CAD build for the part. Positions are in the model's coordinates, mm. A direction names the side the tool comes from. Give positions to 0.01 mm unless a question says otherwise; leave off trailing zeros. Loops run counter-clockwise (first coordinate to the right, second up) from the corner with the lowest first, then second, coordinate; pieces in that order, holes last. Notation, with made-up numbers: (74, 30.25) - (114, 30.25) arc R28 cw to (114, 50.25) - close; hole circle Ø11 at (51.5, 25.25). An arc over 180 degrees is marked (long way). Return JSON: item names as keys, results as strings.
from build123d import *

# Parameters (mm, degrees)
SKETCH1_W           = 220
SKETCH1_H           = 220
BOSS_EXTRUDE1_DEPTH = 4.5
SKETCH2_W           = 220
SKETCH2_H           = 135
BOSS_EXTRUDE2_DEPTH = 4
SKETCH3_W           = 150
SKETCH3_H           = 75
BOSS_EXTRUDE3_DEPTH = 45
SKETCH4_W           = 170
SKETCH4_H           = 110
BOSS_EXTRUDE4_DEPTH = 45
SKETCH5_W           = 280
SKETCH5_H           = 220
BOSS_EXTRUDE5_DEPTH = 4.5
SKETCH6_R           = 1.5
CUT_EXTRUDE1_DEPTH  = 10


with BuildPart() as part:
    # Sketch1 → Boss-Extrude1 (new body)
    with BuildSketch(Plane(origin=(0, 0, 0), x_dir=(1, 0, 0), z_dir=(0, 1, 0))):
        with Locations((-18.301886792, -38.490566038)):
            Rectangle(SKETCH1_W, SKETCH1_H)
    extrude(amount=BOSS_EXTRUDE1_DEPTH)

    # Sketch2 → Boss-Extrude2 (add)
    with BuildSketch(Plane(origin=(0, 4.5, 0), x_dir=(1, 0, 0), z_dir=(0, 1, 0))):
        with Locations((-18.301886792, -65.990566038)):
            Rectangle(SKETCH2_W, SKETCH2_H)
    extrude(amount=BOSS_EXTRUDE2_DEPTH)

    # Sketch3 → Boss-Extrude3 (add)
    with BuildSketch(Plane(origin=(0, 4.5, 0), x_dir=(1, 0, 0), z_dir=(0, 1, 0))):
        with Locations((16.698113208, 34.009433962)):
            Rectangle(SKETCH3_W, SKETCH3_H)
    extrude(amount=BOSS_EXTRUDE3_DEPTH)

    # Sketch4 → Boss-Extrude4 (add)
    with BuildSketch(Plane(origin=(0, 8.5, 0), x_dir=(1, 0, 0), z_dir=(0, 1, 0))):
        with Locations((6.698113208, -63.490566038)):
            Rectangle(SKETCH4_W, SKETCH4_H)
    extrude(amount=BOSS_EXTRUDE4_DEPTH)

    # Sketch5 → Boss-Extrude5 (add)
    with BuildSketch(Plane.XZ):
        with Locations((-48.301886792, 38.490566038)):
            Rectangle(SKETCH5_W, SKETCH5_H)
    extrude(amount=BOSS_EXTRUDE5_DEPTH)

    # Sketch6 → Cut-Extrude1 (cut)
    with BuildSketch(Plane(origin=(0, 0, 0), x_dir=(1, 0, 0), z_dir=(0, 1, 0))):
        with Locations(Location((-168.301886792, 61.509433962, 0), (0, 0, 270))):
            Circle(SKETCH6_R)
        with Locations(Location((-168.301886792, -138.490566038, 0), (0, 0, 270))):
            Circle(SKETCH6_R)
    extrude(amount=-CUT_EXTRUDE1_DEPTH, mode=Mode.SUBTRACT)


solid = part.part
1. Cut at C-C, the plane x = -17.5. Write the cut outline in (y, z).
Values follow:
{"outline": "(-4.5, -71.51) - (49.5, -71.51) - (49.5, 3.49) - (8.5, 3.49) - (8.5, 8.49) - (53.5, 8.49) - (53.5, 118.49) - (8.5, 118.49) - (8.5, 133.49) - (4.5, 133.49) - (4.5, 148.49) - (-4.5, 148.49) - close"}
2. Which spindle directions (+Z, -Z, +X, -X, +Y, -Y) get a long thin tool onto all of the face, cutting with end or side? Do faces 1 (the face through (16, 49.5, -35)), 2 (the face through (-94, 4.5, -37)), 3 (the face through (-128.302, 3, 40)). Say none if no direction does.
Values follow:
{"face 1": "-Z, +X, -X, +Y", "face 2": "-Z, -X, +Y", "face 3": "+Z, -Z, -X, +Y"}
3. Drop flat-ended pins along their axis: P1, Ø4, axis at y = 33.5, z = 111.5, coming from the -X side; P2, Ø6, axis at x = 22, y = 28.5, coming from the +Z side; P3, Ø3.5, axis at x = -168.3, z = 138.49, coming from the +Y side; P4, Ø2.5, axis at x = -168.3, z = -61.51, coming from the -Y side. Give the stop position or say it passes through.
Values follow:
{"P1": "stops at x = -78.3", "P2": "stops at z = 118.49", "P3": "stops at y = 0", "P4": "passes through"}
4. Pull direction Z, two halves, no side cores. Call faces 4 (the face through (12, 23, -71.509)), 5 (the face through (-58.302, 27, -33)), 6 (the face through (6, 31, 8.491)): +Z half, -Z half, draft (parallel to the pull), parting line (faces both ways), or undercut.
Values follow:
{"face 4": "-Z half", "face 5": "draft", "face 6": "undercut"}
5. Cut at B-B, the plane z = 115.5. Write the cut outline in (x, y).
Values follow:
{"outline": "(-188.3, -4.5) - (91.7, -4.5) - (91.7, 53.5) - (-78.3, 53.5) - (-78.3, 8.5) - (-128.3, 8.5) - (-128.3, 0) - (-188.3, 0) - close"}
6. Drill centre lines: probe 1 along Z at (x, y) = (42, 38.5); probe 2 along X at (y, z) = (30, -48); probe 3 along Y at (x, z) = (-107.5, 84). Where is each one in solid material? Low to high.
Values follow:
{"probe 1": "z = -71.51 to 3.49, 8.49 to 118.49", "probe 2": "x = -58.3 to 91.7", "probe 3": "y = -4.5 to 8.5"}
7. Cut at A-A, the plane y = 17.5. Write the cut outline in (x, z).
Values follow:
{"outline": "(-78.3, 8.49) - (91.7, 8.49) - (91.7, 118.49) - (-78.3, 118.49) - close; (-58.3, -71.51) - (91.7, -71.51) - (91.7, 3.49) - (-58.3, 3.49) - close"}
